Build history of the part. All positions in model axes, mm. Face numbers are marked on the shaded views. A direction names the side the tool comes from. Round coordinates to 2 decimals unless told otherwise and drop trailing zeros. Order: outer loops, then holes, each group sorted by start corner. A loop starts at its lowest first (then second) coordinate and runs counter-clockwise, first axis right, second up. Notation, with made-up numbers: (87, -34.5) -> (100, -34.5) arc R26 ccw to (100, -13.5) -> close; hole circle Ø4 at (16.5, -20.5). An arc over 180 degrees is marked (long way). Answer as CSV lines item,"result". Start each with the question number.
```python
from build123d import *

# Parameters (mm, degrees)
F1_DEPTH = 12.7


with BuildPart() as f1:
    # F0 (on Top) → F1 (new body)
    with BuildSketch(Plane.XY):
        with BuildLine():
            Line((-19.05, 12.7), (-19.05, -12.7))
            Line((-19.05, -12.7), (19.05, -12.7))
            Line((19.05, -12.7), (19.05, -3.175))
            Line((19.05, -3.175), (-5.159375, -3.175))
            ThreePointArc((-5.159375, -3.175), (-7.1918990114, -4.0168990114), (-6.35, -1.984375))
            Line((-6.35, -1.984375), (-6.35, 3.175))
            ThreePointArc((-6.35, 3.175), (-10.0319970522, 7.4955975212), (-12.2989024476, 12.7))
            Line((-12.2989024476, 12.7), (-19.05, 12.7))
        make_face()
        with BuildLine():
            Line((-11.4711365721, 12.7), (-12.2989024476, 12.7))
            ThreePointArc((-12.2989024476, 12.7), (-10.0319970522, 7.4955975212), (-6.35, 3.175))
            Line((-6.35, 3.175), (-5.0999496165, 3.175))
            ThreePointArc((-5.0999496165, 3.175), (-9.0409235562, 7.4322327931), (-11.4711365721, 12.7))
        make_face()
        with BuildLine():
            Line((19.05, 12.7), (-11.4711365721, 12.7))
            ThreePointArc((-11.4711365721, 12.7), (-9.0409235562, 7.4322327931), (-5.0999496165, 3.175))
            Line((-5.0999496165, 3.175), (17.7999496165, 3.175))
            ThreePointArc((17.7999496165, 3.175), (18.4369792221, 3.6996313607), (19.05, 4.2521259842))
            Line((19.05, 4.2521259842), (19.05, 12.7))
        make_face()
        with BuildLine():
            Line((17.7999496165, 3.175), (19.05, 3.175))
            Line((19.05, 3.175), (19.05, 4.2521259842))
            ThreePointArc((19.05, 4.2521259842), (18.4369792221, 3.6996313607), (17.7999496165, 3.175))
        make_face()
        with BuildLine():
            ThreePointArc((-6.35, 3.175), (6.35, -1.5875), (19.05, 3.175))
            Line((19.05, 3.175), (17.7999496165, 3.175))
            ThreePointArc((17.7999496165, 3.175), (6.35, -0.7895166667), (-5.0999496165, 3.175))
            Line((-5.0999496165, 3.175), (-6.35, 3.175))
        make_face()
    extrude(amount=F1_DEPTH)


solid = f1.part
```
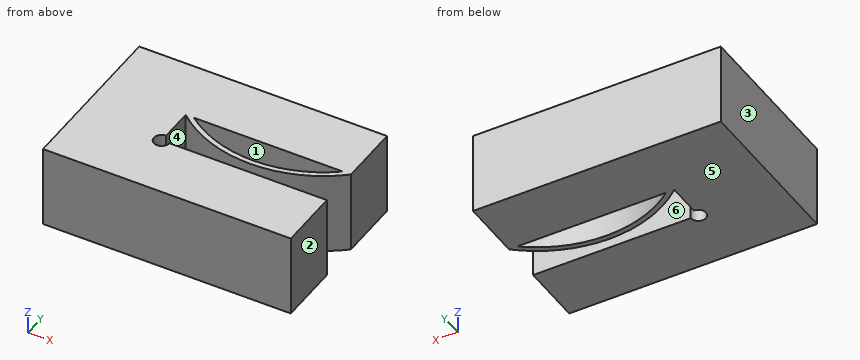
Q1. Probe L1, parallel to Y at x = 7.5, z = 3.5 (3 decimals); L2, parallel to X at y = 2, z = 5; L3, parallel to Y at x = 0.5, z = 12 (3 decimals). List the from-to ranges inside material, lowest first.
Q2. Which spindle directions (+Z, -Z, +X, -X, +Y, -Y) get a long thin tool onto all of the face, cutting with end or side? Do the marked faces 4, 5 and 6. Say none if no direction does.
Q3. Two-plate mould, pull along X, no slides. Class the marked faces 1, 2 and 3: +X half, -X half, draft (parallel to the pull), parting line (faces both ways), or undercut.
Q4. Slice it at C-C, the plane y = 0.5. Write the cut outline in (x, z).
Q5. Slice it at B-B, the plane x = 4. Write the cut outline in (y, z) (3 decimals), plus the area to 3 significant figures.
Q6. Slice it at A-A, the plane z = 8.5. Write the cut outline in (x, y) (3 decimals), plus the area to 3 significant figures.
Q7. Slice it at D-D, the plane y = -3.75. Write the cut outline in (x, z).
Solutions:
1,L1,"y = -12.7 to -3.175, -1.553 to -0.754, 3.175 to 12.7"
1,L2,"x = -19.05 to -6.35, -4.86 to -3.42, 16.12 to 17.56"
1,L3,"y = -12.7 to -3.175, -0.68 to 0.159, 3.175 to 12.7"
2,face 4,"+Z, -Z"
2,face 5,"-Z, +X, -X, +Y, -Y"
2,face 6,"+Z, -Z, +X"
3,face 1,"undercut"
3,face 2,"+X half"
3,face 3,"-X half"
4,outline,"(-19.05, 0) -> (-6.35, 0) -> (-6.35, 12.7) -> (-19.05, 12.7) -> close; (-2.38, 0) -> (-0.44, 0) -> (-0.44, 12.7) -> (-2.38, 12.7) -> close; (13.14, 0) -> (15.08, 0) -> (15.08, 12.7) -> (13.14, 12.7) -> close"
5,outline,"(-12.7, 0) -> (-3.175, 0) -> (-3.175, 12.7) -> (-12.7, 12.7) -> close; (-1.444, 0) -> (-0.64, 0) -> (-0.64, 12.7) -> (-1.444, 12.7) -> close; (3.175, 0) -> (12.7, 0) -> (12.7, 12.7) -> (3.175, 12.7) -> close"
5,area,"252 mm2"
6,outline,"(-19.05, -12.7) -> (19.05, -12.7) -> (19.05, -3.175) -> (-5.159, -3.175) arc R1.191 cw (long way) to (-6.35, -1.984) -> (-6.35, 3.175) arc R19.315 ccw to (19.05, 3.175) -> (19.05, 12.7) -> (-19.05, 12.7) -> close; hole (-5.1, 3.175) arc R18.517 ccw to (17.8, 3.175) -> close"
6,area,"824 mm2"
7,outline,"(-19.05, 0) -> (-7.39, 0) -> (-7.39, 12.7) -> (-19.05, 12.7) -> close; (-5.31, 0) -> (19.05, 0) -> (19.05, 12.7) -> (-5.31, 12.7) -> close"
